Check sheet for the modelled part. Datum: model origin and axes. Units: mm. Face numbers are marked on the shaded views. A direction names the side the tool comes from. Round coordinates to 2 decimals unless told otherwise and drop trailing zeros. Loops run counter-clockwise (first coordinate to the right, second up) from the corner with the lowest first, then second, coordinate; pieces in that order, holes last. Notation, with made-up numbers: (-27.75, -14) -> (7.25, -14) arc R24 ccw to (7.25, 7) -> close; hole circle Ø7 at (-14.5, 47). An arc over 180 degrees is marked (long way). One line per item, written item: value. Start each with the question number.
1. Material ranges on L1, parallel to X at y = 126.5, z = 67.5; L2, parallel to Y at x = 210, z = 58.5; L3, parallel to Y at x = 16, z = 83.5, recorded low to high.
2. Go/stop test with flat-tipped pins: pin 1 (12 mm diameter, centred on x = 252.5, z = 69, fed in from -Y); pin 2 (3 mm diameter, centred on x = 287, z = 26.5, fed in from +Y). Record where each tip stops, or that it passes through.
3. Release check for a two-part mould opening along X. For the marked faces 3, 4 and 5 record: +X half, -X half, draft (parallel to the pull), parting line (faces both ways), or undercut.
4. Cross-section at D-D on x = 340. Record the cut outline in (y, z).
5. Cross-section at A-A on z = 42. Record the cut outline in (x, y).
6. Cross-section at B-B on y = 107. Record the cut outline in (x, z) (3 decimals).
7. Cross-section at C-C on z = 22. Record the cut outline in (x, y).
8. Set-up check for the marked faces 1 and 2: record each of +Z, -Z, +X, -X, +Y, -Y from which the full face is reachable in a straight line by a thin tool's end or side.
from build123d import *

# Parameters (mm, degrees)
BOSS_EXTRUDE1_DEPTH = 100
FILLET4_R           = 50
SKETCH5_R           = 20
CUT_EXTRUDE1_DEPTH  = 421.594816896


with BuildPart() as part:
    # Sketch2 → Boss-Extrude1 (new body)
    with BuildSketch(Plane.XY):
        Polygon((0, 0), (0, 150), (20, 150), (20, 50), (360, 50), (360, 150), (380, 150), (380, 0), align=None)
    extrude(amount=BOSS_EXTRUDE1_DEPTH)

    # Fillet4
    fillet4_edges = [part.edges().sort_by_distance(p)[0] for p in [
        (10, 150, 0),
        (10, 150, 100),
        (370, 150, 100),
        (370, 150, 0),
    ]]
    fillet(fillet4_edges, radius=FILLET4_R - 0.0001)  # a hair under: the kernel refuses the full size

    # Sketch5 → Cut-Extrude1 (cut, through all)
    with BuildSketch(Plane(origin=(380, 0, 0), x_dir=(0, 0, -1), z_dir=(1, 0, 0))):
        with Locations((-50, 100)):
            Circle(SKETCH5_R)
    extrude(amount=-CUT_EXTRUDE1_DEPTH, mode=Mode.SUBTRACT)


solid = part.part
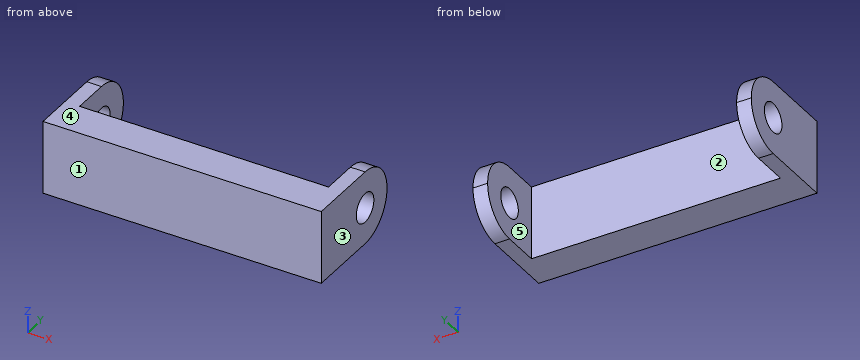
Taken from the geometry:
1. L1: x = 0 to 20, 360 to 380
1. L2: y = 0 to 50
1. L3: y = 0 to 137.12
2. pin 1: stops at y = 0
2. pin 2: stops at y = 50
3. face 3: +X half
3. face 4: draft
3. face 5: undercut
4. outline: (0, 0) -> (50, 0) -> (50, 100) -> (0, 100) -> close
5. outline: (0, 0) -> (380, 0) -> (380, 81.67) -> (360, 81.67) -> (360, 50) -> (20, 50) -> (20, 81.67) -> (0, 81.67) -> close; (0, 118.33) -> (20, 118.33) -> (20, 149.36) -> (0, 149.36) -> close; (360, 118.33) -> (380, 118.33) -> (380, 149.36) -> (360, 149.36) -> close
6. outline: (0, 0.492) -> (20, 0.492) -> (20, 31.265) -> (0, 31.265) -> close; (0, 68.735) -> (20, 68.735) -> (20, 99.508) -> (0, 99.508) -> close; (360, 0.492) -> (380, 0.492) -> (380, 31.265) -> (360, 31.265) -> close; (360, 68.735) -> (380, 68.735) -> (380, 99.508) -> (360, 99.508) -> close
7. outline: (0, 0) -> (380, 0) -> (380, 141.42) -> (360, 141.42) -> (360, 50) -> (20, 50) -> (20, 141.42) -> (0, 141.42) -> close
8. face 1: +Z, -Z, +X, -X, -Y
8. face 2: +Z, -Z, +Y
